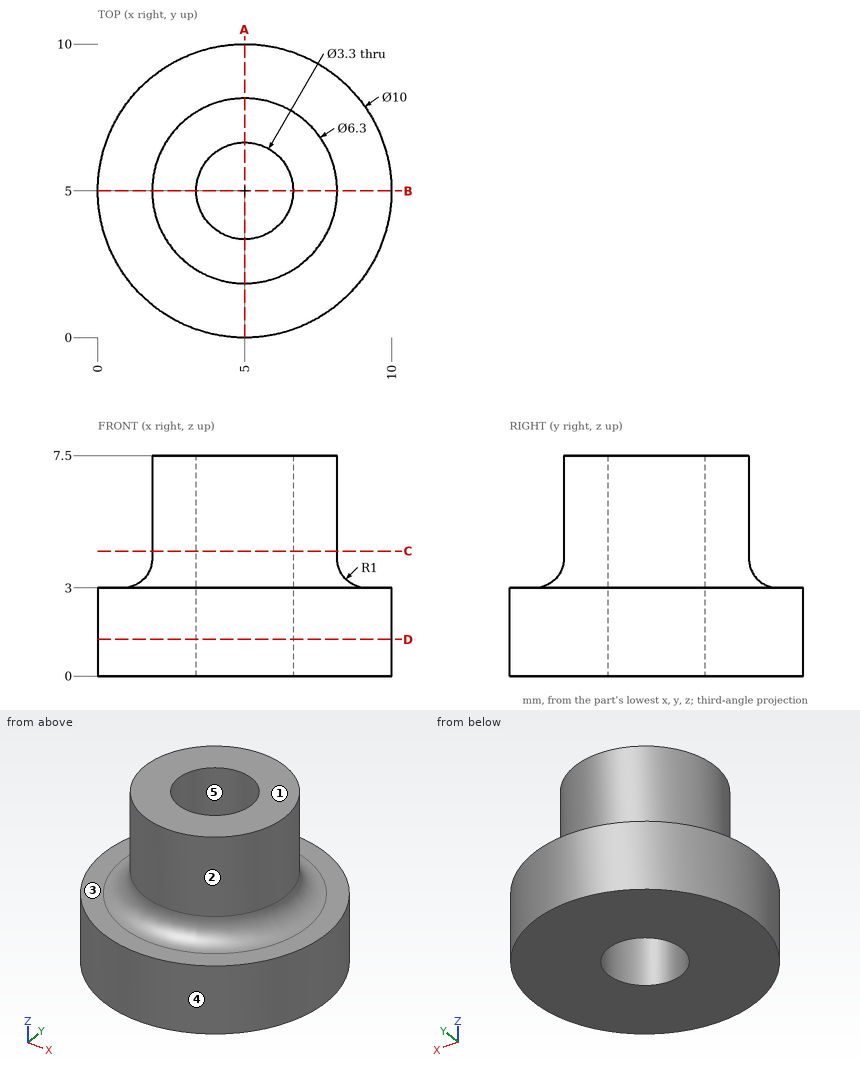
Design review of the part shown in the three views and the two pictorial views. Dimensions are in mm from the part's minimum x, y and z. A direction names the side the tool comes from. Give positions to 0.01 mm unless a question says otherwise; leave off trailing zeros. Loops run counter-clockwise (first coordinate to the right, second up) from the corner with the lowest first, then second, coordinate; pieces in that order, holes last. Notation, with made-up numbers: (-11.5, 28) -> (33.5, 28) arc R28 cw to (33.5, 59) -> close; hole circle Ø11 at (9, 36). An arc over 180 degrees is marked (long way). Write each question's results on one line, items separated by ' | '.
Q1. Machinability: for the marked faces 1 and 2, which of the approach directions +Z, -Z, +X, -X, +Y, -Y give a long, thin tool a straight path to every point of the face, cutting with its end or side? Answer none if there is none.
Reply:
face 1: +Z, +X, -X, +Y, -Y | face 2: +Z
Q2. The part is to be moulded in two halves that separate along X. For the marked faces 3, 4 and 5, say which applies: +X half, -X half, draft (parallel to the pull), parting line (faces both ways), or undercut.
Reply:
face 3: draft | face 4: parting line | face 5: undercut
Q3. Take a section at C-C, the plane z = 4.25. Write out the cut boundary in (x, y), plus the area to 3 significant figures.
Reply:
outline: circle Ø6.3 at (5, 5); hole circle Ø3.3 at (5, 5) | area: 22.6 mm²
Q4. For pin 1 Ø6 at (x, y) = (9, 7) entering from -Z; pin 2 Ø4 at (x, z) = (7.5, 2.5) entering from +Y, all flat-tipped, find the tip position at first contact; note any pin that passes through.
Reply:
pin 1: stops at z = 0 | pin 2: stops at y = 9.97
Q5. Wall thickness on L1, parallel to Y at x = 5, z = 2.75; L2, parallel to Y at x = 5, z = 5.25; L3, parallel to Z at x = 1.25, y = 3.25: over which ranges is each line inside the solid? List them lowest first.
Reply:
L1: y = 0 to 3.35, 6.65 to 10 | L2: y = 1.85 to 3.35, 6.65 to 8.15 | L3: z = 0 to 3
Q6. Take a section at A-A, the plane x = 5. Write out the cut boundary in (y, z), plus the area to 3 significant figures.
Reply:
outline: (0, 0) -> (3.35, 0) -> (3.35, 7.5) -> (1.85, 7.5) -> (1.85, 4) arc R1 cw to (0.85, 3) -> (0, 3) -> close; (6.65, 0) -> (10, 0) -> (10, 3) -> (9.15, 3) arc R1 cw to (8.15, 4) -> (8.15, 7.5) -> (6.65, 7.5) -> close | area: 34.0 mm²
Q7. Take a section at D-D, the plane z = 1.25. Write out the cut boundary in (x, y).
Reply:
outline: circle Ø10 at (5, 5); hole circle Ø3.3 at (5, 5)
